Input: part model. Units: mm. Frame: model coordinates. A direction names the side the tool comes from. Give positions to 0.01 mm unless a question says otherwise; leave off trailing zeros. Write each loop counter-clockwise with the first axis right and the second up, starting at its lowest first coordinate (ties: lowest second). Pieces come first, ordered by that corner, then holes. Notation, with made-up numbers: (85, 39) - (122, 39) arc R24 ccw to (122, 66) - close; hole circle Ø11 at (69.5, 64). An arc over 180 degrees is marked (long way). Use a Markdown table: item, result. Add a question column.
1. Section query D-D, the plane x = 57.5. Return loops of the section in (y, z).
2. Mould query, pull axis X, two halves, no side actions, for faces 1 (the flat face through (75, 1.6, 0.7)), 2 (the cylindrical face through (58.423, 2.958, -35.274)), 3 (the flat face through (-75, 1.6, -0.7)). Classes: released by +X, released by -X, zero draft, split by the parting line, or undercut.
3. Section query C-C, the plane z = 26. Return loops of the section in (x, y).
4. Pin query (flat end, axial travel): pin 1 (3 mm diameter, centred on x = -57.5, z = 33.5, fed in from -Y); pin 2 (1.6 mm diameter, centred on x = 16.5, y = 1.5, fed in from +Z); pin 3 (1 mm diameter, centred on x = -41, y = 4.5, fed in from +Z); pin 4 (2 mm diameter, centred on x = -5.5, y = 0.5, fed in from -Z). Return the tip coordinate at first contact, or that it passes through.
5. Material intervals for probe 1 along Z at (x, y) = (-57.5, 1.85); probe 2 along X at (y, z) = (3.95, -33.5); probe 3 along X at (y, z) = (4.45, -27), sorted ascending.
6. Section query B-B, the plane z = -33.5. Return loops of the section in (x, y).
7. Set-up query: faces 4 (the flat face through (1, 2, 0)), 5 (the cylindrical face through (58.423, 2.958, 31.726)), 6 (the flat face through (40, 2, 33)), 7 (the flat face through (40, 2, -33)). Return all of +Z, -Z, +X, -X, +Y, -Y with unobstructed straight access to the full face (end or side cutting, diameter ignored); none if empty.
8. Section query A-A, the plane y = 0.9. Return loops of the section in (x, z), plus the area to 3 significant figures.
Autodesk Inventor part; units mm, degrees
ref_plane "YZ Plane" through (0, 0, 0) normal (1, 0, 0) x (0, 1, 0)
ref_plane "XZ Plane" through (0, 0, 0) normal (0, 1, 0) x (-1, 0, 0)
ref_plane "XY Plane" through (0, 0, 0) normal (0, 0, 1) x (1, 0, 0)
sketch "Main Base Sketch" plane through (0, 0, 0) normal (0, 1, 0) x (-1, 0, 0)
  line L0 (75, -47) -> (75, 47)
  line L1 (-75, 47) -> (-75, -47)
  line L2 (-75, -47) -> (75, 47) construction
  line L3 (75, -47) -> (-75, 47) construction
  line L4 (-40, -47) -> (-40, -19)
  line L5 (-40, -19) -> (40, -19)
  line L6 (40, -19) -> (40, -47)
  line L7 (40, 19) -> (40, 47)
  line L8 (-40, 19) -> (40, 19)
  line L9 (-40, 47) -> (-40, 19)
  line L10 (75, 47) -> (40, 47)
  line L11 (-40, 47) -> (-75, 47)
  line L12 (-75, -47) -> (-40, -47)
  line L13 (40, -47) -> (75, -47)
  point P0 (0, 0)
  point P1 (0, 0)
  dimension "d0" = 94
  dimension "d1" = 35
  dimension "d2" = 35
  dimension "d3" = 80
  dimension "d4" = 150
  dimension "d5" = 28
  dimension "d6" = 94
  dimension "d8" = 80
  dimension "d9" = 28
  dimension "d27" = 28
  dimension "d28" = 38
  dimension "d37" = 0
extrude "Main Base Extrusion" add sketch "Main Base Sketch" along normal blind 6
sketch "Middle Cut Sketch" plane through (0, 6, 0) normal (0, 1, 0) x (1, 0, 0)
  line L0 (-75, 47) -> (-75, -47)
  line L1 (75, 19) -> (-75, 19)
  line L2 (-75, 19) -> (-75, -19)
  line L3 (-75, -19) -> (75, -19)
  line L4 (75, -19) -> (75, 19)
  line L5 (-40, -19) -> (40, -19)
  line L6 (75, -47) -> (75, 47)
  line L7 (40, 19) -> (-40, 19)
  point P0 (0, 0)
  dimension "d18" = 0
  dimension "d19" = 0
  dimension "d34" = 0
extrude "Middle Cut" cut sketch "Middle Cut Sketch" against normal blind 4
sketch "Arc Sketch" plane through (75, 0, 47) normal (1, 0, 0) x (0, 0, -1)
  line L0 (27, 9.4354) -> (27, -6.3008)
  line L1 (13.5, 8.8022) -> (13.5, -9.7521)
  line L2 (-4.6363, 2) -> (37.5698, 2)
  line L3 (94, 0) -> (0, 0)
  arc A0 (27, 2) -> (0, 2) centre (13.5, -18.7813) ccw
  line L4 (0, 7.9962) -> (0, -1.9448)
  line L5 (0, 0) -> (0, 6)
  line L6 (0, 6) -> (0, 2)
  line L7 (28, 6) -> (0, 6)
  line L8 (0, 6) -> (28, 6)
  line L9 (28, 2) -> (28, 6)
  line L10 (28, 6) -> (28, 2)
  line L11 (28, 2) -> (27, 2)
  line L12 (94, 0) -> (94, 6)
  dimension "d25" = 13.5
  dimension "d26" = 2
  dimension "d29" = 13.5
  dimension "d30" = 27
extrude "Arc Cut" cut sketch "Arc Sketch" against normal through all contours L7 L9 L2 L0 | L0 A0 L7 | A0 L4 L7
mirror "Arc Mirror" about plane through (0, 0, 0) normal (0, 0, 1) of "Arc Cut"
sketch "Arc Holes Sketch" plane through (0, 0, 0) normal (0, -1, 0) x (1, 0, 0)
  circle A0 centre (57.5, 33.5) radius 2
  line L0 (75, -47) -> (75, 47)
  line L1 (40, 47) -> (40, 19)
  line L2 (40, 19) -> (-40, 19)
  line L3 (75, 47) -> (40, 47)
  line L4 (104.495, 0) -> (-129.4816, 0)
  line L5 (0, -57.7002) -> (0, 85.929)
  circle A1 centre (57.5, -33.5) radius 2
  circle A2 centre (-57.5, 33.5) radius 2
  circle A3 centre (-57.5, -33.5) radius 2
  point P0 (0, 0)
  dimension "d38" = 4
  dimension "d39" = 17.5
  dimension "d40" = 17.5
  dimension "d41" = 14.5
  dimension "d42" = 13.5
extrude "Arc Holes Cut" cut sketch "Arc Holes Sketch" against normal through all contours A0 | A1 | A2 | A3
properties part number "TapeMeasureBracketTop"
Result sheet:
| question | item | result |
|---|---|---|
| 1 | outline | (0, -47) - (2, -47) arc R24.78 ccw to (5.92, -35.5) - (0, -35.5) - close; (0, -31.5) - (5.92, -31.5) arc R24.78 ccw to (2, -20) - (2, 20) arc R24.78 ccw to (5.92, 31.5) - (0, 31.5) - close; (0, 35.5) - (5.92, 35.5) arc R24.78 ccw to (2, 47) - (0, 47) - close |
| 2 | face 1 | released by +X |
| 2 | face 2 | undercut |
| 2 | face 3 | released by -X |
| 3 | outline | (-75, 0) - (-40, 0) - (-40, 4.84) - (-75, 4.84) - close; (40, 0) - (75, 0) - (75, 4.84) - (40, 4.84) - close |
| 4 | pin 1 | passes through |
| 4 | pin 2 | stops at z = 19 |
| 4 | pin 3 | stops at z = 43.25 |
| 4 | pin 4 | stops at z = -19 |
| 5 | probe 1 | z = -47 to -35.5, -31.5 to 31.5, 35.5 to 47 |
| 5 | probe 2 | x = -75 to -59.5, -55.5 to -40, 40 to 55.5, 59.5 to 75 |
| 5 | probe 3 | x = -75 to -40, 40 to 75 |
| 6 | outline | (-75, 0) - (-59.5, 0) - (-59.5, 6) - (-75, 6) - close; (-55.5, 0) - (-40, 0) - (-40, 6) - (-55.5, 6) - close; (40, 0) - (55.5, 0) - (55.5, 6) - (40, 6) - close; (59.5, 0) - (75, 0) - (75, 6) - (59.5, 6) - close |
| 7 | face 4 | +X, -X, +Y |
| 7 | face 5 | +Y, -Y |
| 7 | face 6 | +Z, +Y, -Y |
| 7 | face 7 | -Z, +Y, -Y |
| 8 | outline | (-75, -47) - (-40, -47) - (-40, -19) - (40, -19) - (40, -47) - (75, -47) - (75, 47) - (40, 47) - (40, 19) - (-40, 19) - (-40, 47) - (-75, 47) - close; hole circle Ø4 at (-57.5, -33.5); hole circle Ø4 at (-57.5, 33.5); hole circle Ø4 at (57.5, -33.5); hole circle Ø4 at (57.5, 33.5) |
| 8 | area | 9,570 mm² |
